from build123d import *

# Parameters (mm, degrees)
F0_R          = 11
F0_R_2        = 1.5
F0_R_3        = 4
F1_DEPTH      = 3.5
F2_R          = 5
F2_R_2        = 4
F3_DEPTH      = 11
F3_DEPTH_BACK = 5


with BuildPart() as f1:
    # F0 (on Top) → F1 (new body)
    with BuildSketch(Plane.XY):
        Circle(F0_R)
        with Locations((-5.656854, -5.656854)):
            Circle(F0_R_2, mode=Mode.SUBTRACT)
        with Locations((5.656854, -5.656854)):
            Circle(F0_R_2, mode=Mode.SUBTRACT)
        with Locations((-5.656854, 5.656854)):
            Circle(F0_R_2, mode=Mode.SUBTRACT)
        Circle(F0_R_3, mode=Mode.SUBTRACT)
        with Locations((5.656854, 5.656854)):
            Circle(F0_R_2, mode=Mode.SUBTRACT)
    extrude(amount=F1_DEPTH)

    # F2 (on face) → F3 (join, two sides)
    with BuildSketch(Plane(origin=(0, 0, 0), x_dir=(1, 0, 0), z_dir=(0, 0, -1))) as f3_sk:
        Circle(F2_R)
        Circle(F2_R_2, mode=Mode.SUBTRACT)
    extrude(amount=F3_DEPTH)
    extrude(f3_sk.sketch, amount=-F3_DEPTH_BACK)


solid = f1.part
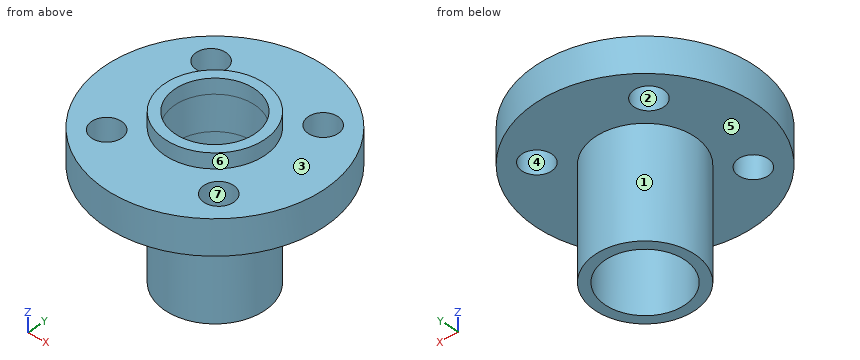
Design review of the part built by this model. Coordinates are the model's own, in mm. Face numbers are marked on the shaded views. A direction names the side the tool comes from. Coordinates: 2 decimals unless noted, no trailing zeros. Write each loop counter-clockwise with the first axis right and the second up, starting at its lowest first coordinate (ties: lowest second). Pieces come first, ordered by that corner, then holes. Notation, with made-up numbers: (31.5, 4.5) - (68.5, 4.5) arc R15 ccw to (68.5, 30.5) - close; hole circle Ø6 at (82, 33). An arc over 180 degrees is marked (long way). One line per item, written item: value.
1) Insertion check: pin 1 (3.5 mm diameter, centred on x = 5.66, y = -5.66, fed in from +Z); pin 2 (6 mm diameter, centred on y = -3, z = -7, fed in from +X); pin 3 (2 mm diameter, centred on y = 5.5, z = -7.5, fed in from +X). Each pin has a flat end and moves straight along its axis. Give the tip position at first contact, or say it passes through.
Answer sheet:
pin 1: stops at z = 3.5
pin 2: stops at x = 5
pin 3: stops at x = 2.18
2) For the marked faces 1, 2 and 3, list the 3-axis set-ups (+Z, -Z, +X, -X, +Y, -Y) from which the entire face can be reached by the end or side of a thin tool; tool diameter is ignored.
Answer sheet:
face 1: -Z
face 2: +Z, -Z
face 3: +Z
3) Add section A-A (y = 0). State the section outline as (x, z) points, plus the area to 3 significant figures.
Answer sheet:
outline: (-11, 0) - (-5, 0) - (-5, -11) - (-4, -11) - (-4, 5) - (-5, 5) - (-5, 3.5) - (-11, 3.5) - close; (4, -11) - (5, -11) - (5, 0) - (11, 0) - (11, 3.5) - (5, 3.5) - (5, 5) - (4, 5) - close
area: 74.0 mm2
4) Add section D-D (x = 6.75). State the section outline as (y, z) points.
Answer sheet:
outline: (-8.69, 0) - (-6.68, 0) - (-6.68, 3.5) - (-8.69, 3.5) - close; (-4.63, 0) - (4.63, 0) - (4.63, 3.5) - (-4.63, 3.5) - close; (6.68, 0) - (8.69, 0) - (8.69, 3.5) - (6.68, 3.5) - close
5) To check wall thickness, follow probe 1 along Y at (x, z) = (0, -3); probe 2 along Z at (x, y) = (-0.25, 8.75). State the ranges of each line that lie inside material, in increasing order.
Answer sheet:
probe 1: y = -5 to -4, 4 to 5
probe 2: z = 0 to 3.5
6) Mouldability with a two-part tool opening along X and no side actions: class the marked faces 4, 5, 6 and 7 as +X half, -X half, draft (parallel to the pull), parting line (faces both ways), or undercut.
Answer sheet:
face 4: undercut
face 5: draft
face 6: parting line
face 7: undercut
7) Add section C-C (z = 1.75). State the section outline as (x, y) points.
Answer sheet:
outline: circle Ø22 at (0, 0); hole circle Ø3 at (-5.66, -5.66); hole circle Ø3 at (-5.66, 5.66); hole circle Ø8 at (0, 0); hole circle Ø3 at (5.66, -5.66); hole circle Ø3 at (5.66, 5.66)
